Autodesk Inventor part; units mm, degrees
ref_plane "YZ Plane" through (0, 0, 0) normal (1, 0, 0) x (0, 1, 0)
ref_plane "XZ Plane" through (0, 0, 0) normal (0, 1, 0) x (-1, 0, 0)
ref_plane "XY Plane" through (0, 0, 0) normal (0, 0, 1) x (1, 0, 0)
sketch "Sketch1" plane through (0, 0, 0) normal (0, 1, 0) x (-1, 0, 0)
  circle A0 centre (0, 0) radius 7.5
  dimension "d0" = 15
extrude "Extrusion1" add sketch "Sketch1" along normal blind 8
sketch "Sketch2" plane through (0, 8, 0) normal (0, 1, 0) x (1, 0, 0)
  circle A0 centre (0, 0) radius 7.5
  circle A1 centre (0, 0) radius 5
  dimension "d3" = 10
extrude "Extrusion2" add sketch "Sketch2" along normal blind 5 contours A1
sketch "Sketch3" plane through (0, 13, 0) normal (0, 1, 0) x (1, 0, 0)
  circle A0 centre (0, 0) radius 5
  circle A1 centre (0, 0) radius 3 construction
  line L0 (-2.6295, 1.4442) -> (2.6295, 1.4442)
  arc A2 (-2.6295, 1.4442) -> (2.6295, 1.4442) centre (0, 0) ccw
  dimension "d6" = 6
  dimension "d7" = 5.259
extrude "Extrusion3" cut sketch "Sketch3" against normal blind 11 contours L0 A2
chamfer "Chamfer1" distance 1 angle 45 1 edges at (7.5, 0, 0)
sketch "Sketch4" plane through (0, 0, 0) normal (0, -1, 0) x (1, 0, 0)
  circle A0 centre (0, 0) radius 6.5 construction
  line L0 (0, 0) -> (0, 6.5) construction
  line L1 (-0.5, 4.5) -> (0.5, 4.5)
  line L2 (0.5, 4.5) -> (0.5, 7.5)
  line L3 (0.5, 7.5) -> (-0.5, 7.5)
  line L4 (-0.5, 7.5) -> (-0.5, 4.5)
  circle A1 centre (0, 0) radius 7.5 construction
  line L5 (-3.0495, 3.3467) -> (-2.2405, 3.9345)
  line L6 (-2.2405, 3.9345) -> (-4.0039, 6.3615)
  line L7 (-4.0039, 6.3615) -> (-4.8129, 5.7737)
  line L8 (-4.8129, 5.7737) -> (-3.0495, 3.3467)
  line L9 (-4.4343, 0.915) -> (-4.1252, 1.8661)
  line L10 (-4.1252, 1.8661) -> (-6.9784, 2.7932)
  line L11 (-6.9784, 2.7932) -> (-7.2874, 1.8421)
  line L12 (-7.2874, 1.8421) -> (-4.4343, 0.915)
  line L13 (-4.1252, -1.8661) -> (-4.4343, -0.915)
  line L14 (-4.4343, -0.915) -> (-7.2874, -1.8421)
  line L15 (-7.2874, -1.8421) -> (-6.9784, -2.7932)
  line L16 (-6.9784, -2.7932) -> (-4.1252, -1.8661)
  line L17 (-2.2405, -3.9345) -> (-3.0495, -3.3467)
  line L18 (-3.0495, -3.3467) -> (-4.8129, -5.7737)
  line L19 (-4.8129, -5.7737) -> (-4.0039, -6.3615)
  line L20 (-4.0039, -6.3615) -> (-2.2405, -3.9345)
  line L21 (0.5, -4.5) -> (-0.5, -4.5)
  line L22 (-0.5, -4.5) -> (-0.5, -7.5)
  line L23 (-0.5, -7.5) -> (0.5, -7.5)
  line L24 (0.5, -7.5) -> (0.5, -4.5)
  line L25 (3.0495, -3.3467) -> (2.2405, -3.9345)
  line L26 (2.2405, -3.9345) -> (4.0039, -6.3615)
  line L27 (4.0039, -6.3615) -> (4.8129, -5.7737)
  line L28 (4.8129, -5.7737) -> (3.0495, -3.3467)
  line L29 (4.4343, -0.915) -> (4.1252, -1.8661)
  line L30 (4.1252, -1.8661) -> (6.9784, -2.7932)
  line L31 (6.9784, -2.7932) -> (7.2874, -1.8421)
  line L32 (7.2874, -1.8421) -> (4.4343, -0.915)
  line L33 (4.1252, 1.8661) -> (4.4343, 0.915)
  line L34 (4.4343, 0.915) -> (7.2874, 1.8421)
  line L35 (7.2874, 1.8421) -> (6.9784, 2.7932)
  line L36 (6.9784, 2.7932) -> (4.1252, 1.8661)
  line L37 (2.2405, 3.9345) -> (3.0495, 3.3467)
  line L38 (3.0495, 3.3467) -> (4.8129, 5.7737)
  line L39 (4.8129, 5.7737) -> (4.0039, 6.3615)
  line L40 (4.0039, 6.3615) -> (2.2405, 3.9345)
  point P0 (0, 4.5)
  point P1 (-2.645, 3.6406)
  point P2 (-4.2798, 1.3906)
  point P3 (-4.2798, -1.3906)
  point P4 (-2.645, -3.6406)
  point P5 (0, -4.5)
  point P6 (2.645, -3.6406)
  point P7 (4.2798, -1.3906)
  point P8 (4.2798, 1.3906)
  point P9 (2.645, 3.6406)
  dimension "d13" = 1
  dimension "d14" = 3
  dimension "d17" = 360
extrude "Extrusion4" cut sketch "Sketch4" against normal blind 0.5
properties part number "rotary_encoder_cnob" material "ABS Plastic"
For this review, take the finished solid that the model builds, in its own axes (mm). A direction names the side the tool comes from. Round coordinates to 2 decimals unless told otherwise and drop trailing zeros. Write each loop counter-clockwise with the first axis right and the second up, starting at its lowest first coordinate (ties: lowest second). Pieces come first, ordered by that corner, then holes. Notation, with made-up numbers: (70.25, -13) -> (82.25, -13) arc R21 cw to (82.25, 20) -> close; hole circle Ø5 at (6, 72.5). An arc over 180 degrees is marked (long way). Use one line per item in the form item = value.
Q1. Consider section D-D (y = 12.25). State the section outline as (x, z) points.
Resolved:
outline = circle Ø10 at (0, 0); hole (-2.63, -1.44) -> (2.63, -1.44) arc R3 ccw (long way) to start
Q2. The part is to be moulded in two halves that separate along X. For faces 1 (the flat face through (2.96, 0.246, -4.924)), 2 (the conical face through (5.3, 0.2, -4.1)), 3 (the flat face through (-2, 8, -5)), say which applies: released by +X, released by -X, zero draft, split by the parting line, or undercut.
Resolved:
face_1 = undercut
face_2 = split by the parting line
face_3 = zero draft
Q3. Consider section A-A (z = 0). State the section outline as (x, y) points.
Resolved:
outline = (-7.5, 1) -> (-6.5, 0) -> (6.5, 0) -> (7.5, 1) -> (7.5, 8) -> (5, 8) -> (5, 13) -> (3, 13) -> (3, 2) -> (-3, 2) -> (-3, 13) -> (-5, 13) -> (-5, 8) -> (-7.5, 8) -> close
Q4. Machinability: for faces 4 (the cylindrical face through (-1.08, 10.46, -4.88)), 5 (the flat face through (-3.789, 0.247, 4.365)), 6 (the flat face through (0, 0.5, 6)), which of the approach directions +Z, -Z, +X, -X, +Y, -Y give a long, thin tool a straight path to every point of the face, cutting with its end or side? Answer none if there is none.
Resolved:
face_4 = +Y
face_5 = -Y
face_6 = +Z, -Y
Q5. Consider section B-B (x = 0). State the section outline as (y, z) points, then the cut area to 3 significant figures.
Resolved:
outline = (0, -4.5) -> (0.5, -4.5) -> (0.5, -7) -> (1, -7.5) -> (8, -7.5) -> (8, -5) -> (13, -5) -> (13, -1.44) -> (2, -1.44) -> (2, 3) -> (13, 3) -> (13, 5) -> (8, 5) -> (8, 7.5) -> (1, 7.5) -> (0.5, 7) -> (0.5, 4.5) -> (0, 4.5) -> close
area = 118 mm²
Q6. Clearance check with flat-ended pins moving along their axes: pin 1 Ø3 at (x, y) = (5.5, 4.5) entering from +Z; pin 2 Ø2 at (x, y) = (-2.5, 3.5) entering from +Z; pin 3 Ø0.7 at (x, z) = (-3.5, 5) entering from -Y. State where each tip first meets the part, or that it passes through.
Resolved:
pin_1 = 6.34
pin_2 = 7.35
pin_3 = 0.5
Q7. To check wall thickness, follow probe 1 along X at (y, z) = (8.75, 0); probe 2 along Z at (x, y) = (0, 8.75); probe 3 along Z at (x, y) = (0, 7.25). State the ranges of each line that lie inside material, in increasing order. Write a range as from..to.
Resolved:
probe_1 = -5..-3, 3..5
probe_2 = -5..-1.44, 3..5
probe_3 = -7.5..-1.44, 3..7.5
Q8. Consider section C-C (y = 3.75). State the section outline as (x, z) points.
Resolved:
outline = circle Ø15 at (0, 0); hole (-2.63, -1.44) -> (2.63, -1.44) arc R3 ccw (long way) to start
